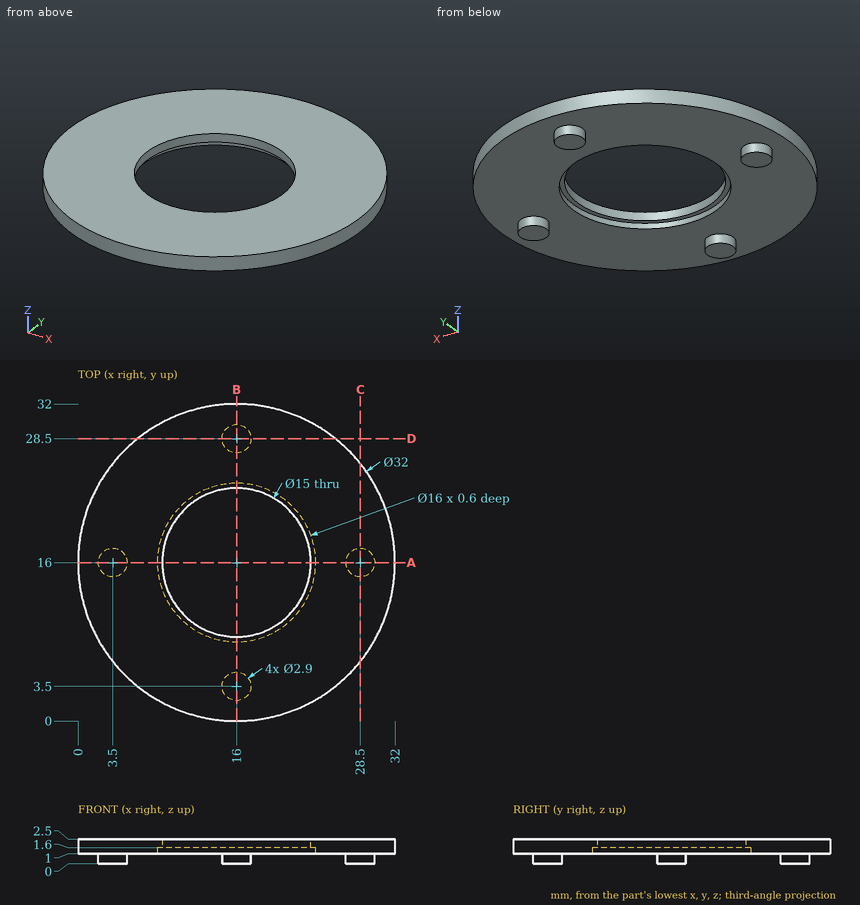
Design review of the part shown in the three views and the two pictorial views. Dimensions are in mm from the part's minimum x, y and z. Round coordinates to 2 decimals unless told otherwise and drop trailing zeros. Write each loop counter-clockwise with the first axis right and the second up, starting at its lowest first coordinate (ties: lowest second). Pieces come first, ordered by that corner, then holes.
Item 1: We need section C-C on x = 28.5. Write out the cut boundary in (y, z), and give its area (3 significant figures).
Item 2: Clearance check with flat-ended pins moving along their axes: pin 1 Ø1.5 at (x, z) = (24, 1) entering from +Y; pin 2 Ø13 at (x, y) = (16, 16) entering from -Z; pin 3 Ø9.5 at (x, y) = (11, 13) entering from -Z. State where each tip first meets the part, or that it passes through.
Item 3: We need section A-A on y = 16. Write out the cut boundary in (x, z), and give its area (3 significant figures).
Item 4: For probe 1 along Z at (x, y) = (14, 4); probe 2 along Z at (x, y) = (9, 19.5); probe 3 along X at (y, z) = (12.5, 2.05), list the stretches that pass through material, from the lowest coordinate up.
Returned:
1. outline: (6.01, 1) - (14.55, 1) - (14.55, 0) - (17.45, 0) - (17.45, 1) - (25.99, 1) - (25.99, 2.5) - (6.01, 2.5) - close
1. area: 32.9 mm2
2. pin 1: stops at y = 30.26
2. pin 2: passes through
2. pin 3: stops at z = 1
3. outline: (0, 1) - (2.05, 1) - (2.05, 0) - (4.95, 0) - (4.95, 1) - (8, 1) - (8, 1.6) - (8.5, 1.6) - (8.5, 2.5) - (0, 2.5) - close; (23.5, 1.6) - (24, 1.6) - (24, 1) - (27.05, 1) - (27.05, 0) - (29.95, 0) - (29.95, 1) - (32, 1) - (32, 2.5) - (23.5, 2.5) - close
3. area: 30.7 mm2
4. probe 1: z = 1 to 2.5
4. probe 2: z = 1.6 to 2.5
4. probe 3: x = 0.39 to 9.37, 22.63 to 31.61
